Could you check a few things on this model? Use its own coordinates, in mm. A direction names the side the tool comes from. Round coordinates to 2 decimals unless told otherwise and drop trailing zeros. Loops run counter-clockwise (first coordinate to the right, second up) from the corner with the lowest first, then second, coordinate; pieces in that order, holes last. Notation, with made-up numbers: (34.5, 67.25) -> (91.5, 67.25) arc R22 ccw to (91.5, 95.25) -> close; hole circle Ø10 at (-7.75, 19.5). An arc over 180 degrees is marked (long way). Put each result on its own line as item: value. Start each with the question number.
1. I need wall thicknesses on line 1 (X direction, y = 1.7, z = 0); line 2 (X direction, y = 2.65, z = 4); line 3 (Z direction, x = 5.5, y = 4.4). Which ranges of each line are inside material? Lowest first, please. Write a range as [from, to].
2. Imagine slicing it at B-B, the plane y = 1.7. Please give me the cut outline in (x, z), and give its area (3 significant figures).
3. If we mould it in two halves opening along X, with no side actions, what happens to faces 1 (the flat face through (-70, 2, -57.5)), 2 (the flat face through (-1, 2, 70)), 3 (the flat face through (-90, 2, 1))? For each: pulls with the +X half, pulls with the -X half, needs draft (parallel to the pull), parting line crosses it, or undercut.
4. Imagine slicing it at C-C, the plane x = 42. Please give me the cut outline in (y, z), and give its area (3 significant figures).
5. Imagine slicing it at A-A, the plane z = 0. Please give me the cut outline in (x, y), and give its area (4 significant figures).
6. Which directions (+Z, -Z, +X, -X, +Y, -Y) give clear straight access to the entire face, cutting with the end or side of a thin tool? Please do faces 4 (the flat face through (-1, 2, -70)), 5 (the flat face through (-75, 2, -55)).
7. I'm going to push a flat-ended pin straight in: P1, Ø5, axis at x = 42, z = -54.9, coming from the -Y side. Where does the tip first touch, or does it pass through?
```python
from build123d import *

# Parameters (mm, degrees)
IZIM1_W                     = 180
IZIM1_H                     = 140
IZIM1_R                     = 14.75
IZIM1_R_2                   = 3
IZIM1_W_2                   = 10
IZIM1_H_2                   = 5
Y_KSEKLIK_EKSTR_ZYON1_DEPTH = 5


with BuildPart() as part:
    # Çizim1 → Yükseklik-Ekstrüzyon1 (new body)
    with BuildSketch(Plane(origin=(0, 0, 0), x_dir=(1, 0, 0), z_dir=(0, 1, 0))):
        Rectangle(IZIM1_W, IZIM1_H)
        with Locations(Location((0, 0, 0), (0, 0, 270))):
            Circle(IZIM1_R, mode=Mode.SUBTRACT)
        with Locations(Location((70, 54.895079595, 0), (0, 0, 270))):
            Circle(IZIM1_R_2, mode=Mode.SUBTRACT)
        with Locations(Location((42, 54.895079595, 0), (0, 0, 270))):
            Circle(IZIM1_R_2, mode=Mode.SUBTRACT)
        with Locations(Location((14, 54.895079595, 0), (0, 0, 270))):
            Circle(IZIM1_R_2, mode=Mode.SUBTRACT)
        with Locations(Location((-14, 54.895079595, 0), (0, 0, 270))):
            Circle(IZIM1_R_2, mode=Mode.SUBTRACT)
        with Locations(Location((-42, 54.895079595, 0), (0, 0, 270))):
            Circle(IZIM1_R_2, mode=Mode.SUBTRACT)
        with Locations((-70, 55)):
            Rectangle(IZIM1_W_2, IZIM1_H_2, mode=Mode.SUBTRACT)
    extrude(amount=Y_KSEKLIK_EKSTR_ZYON1_DEPTH)


solid = part.part
```
Entries:
1. line 1: [-90, -14.75], [14.75, 90]
1. line 2: [-90, -14.2], [14.2, 90]
1. line 3: [-70, -13.69], [13.69, 70]
2. outline: (-90, -70) -> (90, -70) -> (90, 70) -> (-90, 70) -> close; hole (-75, -57.5) -> (-65, -57.5) -> (-65, -52.5) -> (-75, -52.5) -> close; hole circle Ø6 at (-42, -54.9); hole circle Ø6 at (-14, -54.9); hole circle Ø29.5 at (0, 0); hole circle Ø6 at (14, -54.9); hole circle Ø6 at (42, -54.9); hole circle Ø6 at (70, -54.9)
2. area: 24,300 mm^2
3. face 1: undercut
3. face 2: needs draft
3. face 3: pulls with the -X half
4. outline: (0, -70) -> (5, -70) -> (5, -57.9) -> (0, -57.9) -> close; (0, -51.9) -> (5, -51.9) -> (5, 70) -> (0, 70) -> close
4. area: 670 mm^2
5. outline: (-90, 0) -> (-14.75, 0) -> (-14.75, 5) -> (-90, 5) -> close; (14.75, 0) -> (90, 0) -> (90, 5) -> (14.75, 5) -> close
5. area: 752.5 mm^2
6. face 4: -Z, +X, -X, +Y, -Y
6. face 5: +Y, -Y
7. P1: through
